Here's the drawing with two shaded views (mm, measured from the low corner). I have some questions. A direction names the side the tool comes from. Give positions to 0.01 mm unless a question says otherwise; leave off trailing zeros. Write each loop counter-clockwise with the first axis right and the second up, starting at its lowest first coordinate (ties: lowest second). Pieces come first, ordered by that corner, then holes. Notation, with made-up numbers: (16.25, 41.25) - (53.25, 41.25) arc R14 ccw to (53.25, 65.25) - close; hole circle Ø9 at (-18, 73). An arc over 180 degrees is marked (long way). Use one line per item in the form item = value.
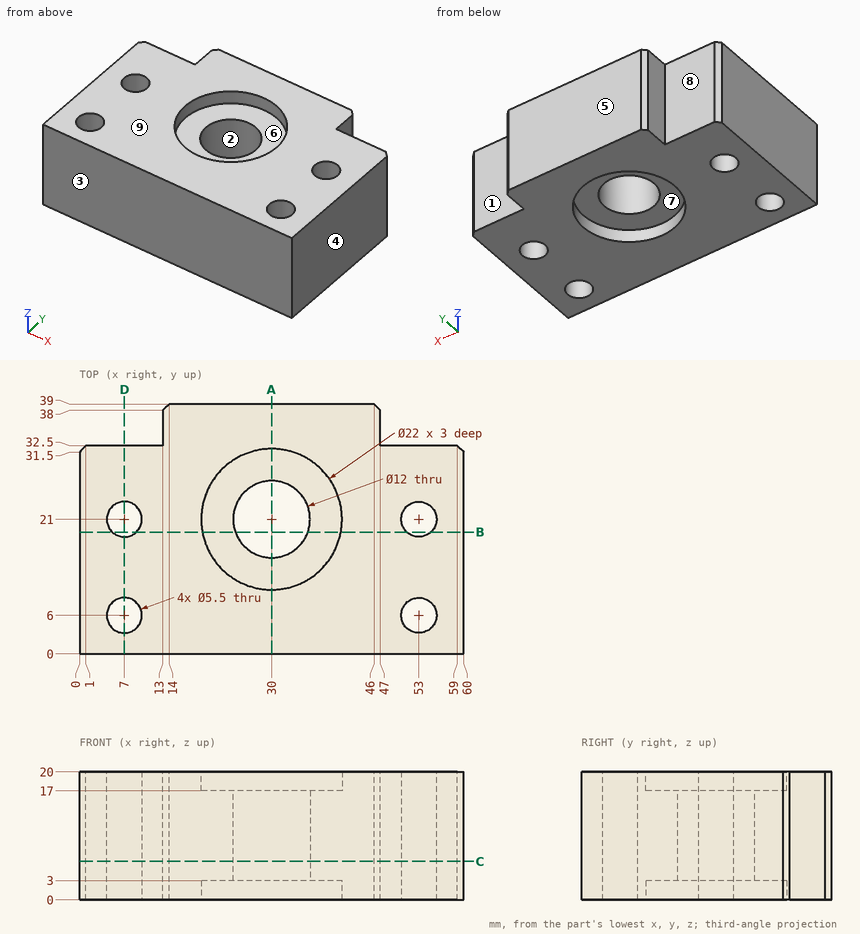
1. Imagine slicing it at C-C, the plane z = 6. List the corners of the cut face in (x, y) for me.
Response values:
outline = (0, 0) - (60, 0) - (60, 31.5) - (59, 32.5) - (47, 32.5) - (47, 38) - (46, 39) - (14, 39) - (13, 38) - (13, 32.5) - (1, 32.5) - (0, 31.5) - close; hole circle Ø5.5 at (7, 6); hole circle Ø5.5 at (7, 21); hole circle Ø12 at (30, 21); hole circle Ø5.5 at (53, 6); hole circle Ø5.5 at (53, 21)
2. If we mould it in two halves opening along Y, with no side actions, what happens to the marked faces 1, 2, 3 and 4? For each: pulls with the +Y half, pulls with the -Y half, needs draft (parallel to the pull), parting line crosses it, or undercut.
Response values:
face_1 = pulls with the +Y half
face_2 = undercut
face_3 = pulls with the -Y half
face_4 = needs draft
3. Imagine slicing it at B-B, the plane y = 19. List the corners of the cut face in (x, z) for me, and give its area (3 significant figures).
Response values:
outline = (0, 0) - (5.11, 0) - (5.11, 20) - (0, 20) - close; (8.89, 0) - (19.18, 0) - (19.18, 3) - (24.34, 3) - (24.34, 17) - (19.18, 17) - (19.18, 20) - (8.89, 20) - close; (35.66, 3) - (40.82, 3) - (40.82, 0) - (51.11, 0) - (51.11, 20) - (40.82, 20) - (40.82, 17) - (35.66, 17) - close; (54.89, 0) - (60, 0) - (60, 20) - (54.89, 20) - close
area = 761 mm²
4. Imagine slicing it at D-D, the plane x = 7. List the corners of the cut face in (y, z) for me.
Response values:
outline = (0, 0) - (3.25, 0) - (3.25, 20) - (0, 20) - close; (8.75, 0) - (18.25, 0) - (18.25, 20) - (8.75, 20) - close; (23.75, 0) - (32.5, 0) - (32.5, 20) - (23.75, 20) - close
5. Which directions (+Z, -Z, +X, -X, +Y, -Y) give clear straight access to the entire face, cutting with the end or side of a thin tool? Please do the marked faces 5, 6, 7, 8 and 9.
Response values:
face_5 = +Z, -Z, +X, -X, +Y
face_6 = +Z
face_7 = -Z
face_8 = +Z, -Z, -X, +Y
face_9 = +Z, +X, -X, +Y, -Y
6. Imagine slicing it at A-A, the plane x = 30. List the corners of the cut face in (y, z) for me.
Response values:
outline = (0, 0) - (10, 0) - (10, 3) - (15, 3) - (15, 17) - (10, 17) - (10, 20) - (0, 20) - close; (27, 3) - (32, 3) - (32, 0) - (39, 0) - (39, 20) - (32, 20) - (32, 17) - (27, 17) - close
7. For pin 1 (3 mm diameter, centred on y = 36, z = 7, fed in from +X); pin 2 (1.5 mm diameter, centred on x = 26.5, y = 28, fed in from -Z); pin 3 (3.5 mm diameter, centred on x = 4.5, z = 7, fed in from +Y), each with a flat end and sliding along its axis, tell me the tip position at first contact or that it passes through.
Response values:
pin_1 = 47
pin_2 = 3
pin_3 = 32.5
8. If I drill on line 1 (Y direction, x = 53, z = 9.75); line 2 (X direction, y = 18.5, z = 10.5); line 3 (X direction, y = 20, z = 18), over which ranges is the centre line in solid material (lowest first)? Write a range as from..to.
Response values:
line_1 = 0..3.25, 8.75..18.25, 23.75..32.5
line_2 = 0..5.85, 8.15..24.55, 35.45..51.85, 54.15..60
line_3 = 0..4.44, 9.56..19.05, 40.95..50.44, 55.56..60
